from build123d import *

# Parameters (mm, degrees)
SKETCH_1_W          = 150
SKETCH_1_H          = 80
EXTRUDE_1_DEPTH     = 3.2
SKETCH_2_R          = 12.5
CUT_EXTRUDE_1_DEPTH = 3.2
SKETCH_3_R          = 1.6
CUT_EXTRUDE_3_DEPTH = 3.2


with BuildPart() as part:
    # 草图1 → 凸台-拉伸1 (new body)
    with BuildSketch(Plane(origin=(0, 0, 0), x_dir=(1, 0, 0), z_dir=(0, 1, 0))):
        Rectangle(SKETCH_1_W, SKETCH_1_H)
    extrude(amount=EXTRUDE_1_DEPTH)

    # 草图2 → 切除-拉伸1 (cut)
    with BuildSketch(Plane(origin=(0, 3.2, 0), x_dir=(1, 0, 0), z_dir=(0, 1, 0))):
        with Locations(Location((0, 0, 0), (0, 0, 270))):
            Circle(SKETCH_2_R)
    extrude(amount=-CUT_EXTRUDE_1_DEPTH, mode=Mode.SUBTRACT)

    # 草图3 → 切除-拉伸3 (cut)
    with BuildSketch(Plane(origin=(0, 3.2, 0), x_dir=(1, 0, 0), z_dir=(0, 1, 0))):
        with Locations(Location((0, -22, 0), (0, 0, 270))):
            Circle(SKETCH_3_R)
        with Locations(Location((-22, 0, 0), (0, 0, 270))):
            Circle(SKETCH_3_R)
        with Locations(Location((0, 22, 0), (0, 0, 270))):
            Circle(SKETCH_3_R)
        with Locations(Location((22, 0, 0), (0, 0, 270))):
            Circle(SKETCH_3_R)
    extrude(amount=-CUT_EXTRUDE_3_DEPTH, mode=Mode.SUBTRACT)


solid = part.part
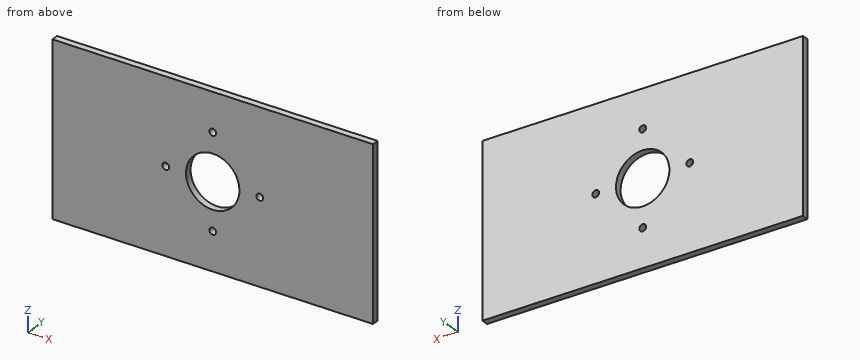
Read the model definition and answer for the solid it produces. Units are mm, in the model's axes. Coordinates: 2 decimals unless noted, no trailing zeros. Loops run counter-clockwise (first coordinate to the right, second up) from the corner with the lowest first, then second, coordinate; pieces in that order, holes last.
Q1. The part is cut by section B-B on z = 0. Write down the section's boundary in (x, y).
Q2. The part is cut by section D-D on z = 22. Write down the section's boundary in (x, y).
Q3. The part is cut by section A-A on x = 0. Write down the section's boundary in (y, z), and give its area (3 significant figures).
Q4. Consider probe 1 along X at (y, z) = (1.95, 0); probe 2 along X at (y, z) = (1.15, 22); probe 3 along Z at (x, y) = (3.5, 3). Determine where each line is inside the solid, lowest interval first.
Q5. The part is cut by section C-C on y = 2. Write down the section's boundary in (x, z), and give its area (3 significant figures).
Results below:
1. outline: (-75, 0) - (-23.6, 0) - (-23.6, 3.2) - (-75, 3.2) - close; (-20.4, 0) - (-12.5, 0) - (-12.5, 3.2) - (-20.4, 3.2) - close; (12.5, 0) - (20.4, 0) - (20.4, 3.2) - (12.5, 3.2) - close; (23.6, 0) - (75, 0) - (75, 3.2) - (23.6, 3.2) - close
2. outline: (-75, 0) - (-1.6, 0) - (-1.6, 3.2) - (-75, 3.2) - close; (1.6, 0) - (75, 0) - (75, 3.2) - (1.6, 3.2) - close
3. outline: (0, -40) - (3.2, -40) - (3.2, -23.6) - (0, -23.6) - close; (0, -20.4) - (3.2, -20.4) - (3.2, -12.5) - (0, -12.5) - close; (0, 12.5) - (3.2, 12.5) - (3.2, 20.4) - (0, 20.4) - close; (0, 23.6) - (3.2, 23.6) - (3.2, 40) - (0, 40) - close
3. area: 156 mm2
4. probe 1: x = -75 to -23.6, -20.4 to -12.5, 12.5 to 20.4, 23.6 to 75
4. probe 2: x = -75 to -1.6, 1.6 to 75
4. probe 3: z = -40 to -12, 12 to 40
5. outline: (-75, -40) - (75, -40) - (75, 40) - (-75, 40) - close; hole circle Ø3.2 at (-22, 0); hole circle Ø25 at (0, 0); hole circle Ø3.2 at (0, -22); hole circle Ø3.2 at (0, 22); hole circle Ø3.2 at (22, 0)
5. area: 11,500 mm2
